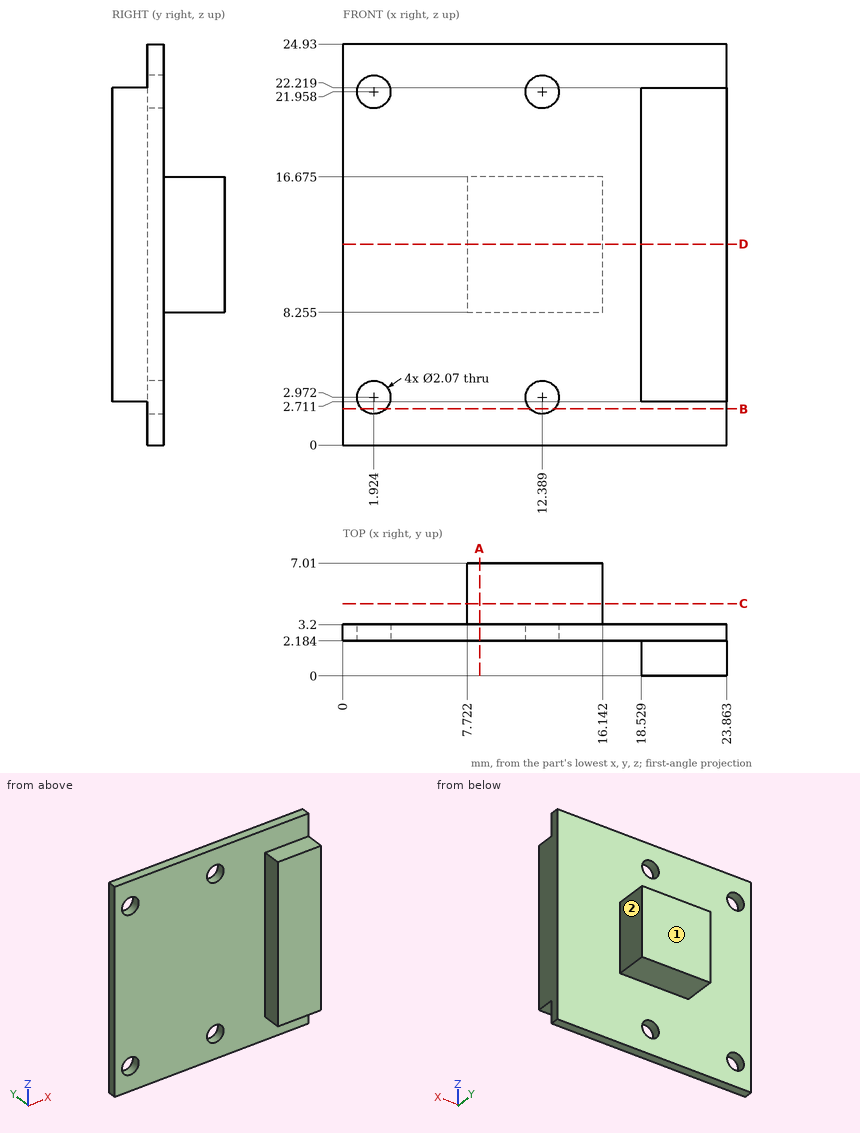
Input: dimensioned drawing with shaded views. Units: mm. Origin: part minimum x, y, z. A direction names the side the tool comes from. Coordinates: 2 decimals unless noted, no trailing zeros. Loops run counter-clockwise (first coordinate to the right, second up) from the corner with the lowest first, then second, coordinate; pieces in that order, holes last. Notation, with made-up numbers: (50.5, 33) -> (104.5, 33) arc R16 cw to (104.5, 45) -> close; hole circle Ø6 at (89.5, 6). An arc over 180 degrees is marked (long way). One line per item, written item: value. Start each with the question number.
Q1. Contact query for flat-ended pins moving along their axis: P1, Ø3, axis at x = 13, y = 5, coming from the +Z side (3 decimals); P2, Ø7, axis at x = 14, z = 8.5, coming from the -Y side; P3, Ø3, axis at y = 5, z = 10.5, coming from the -X side. Output: stop coordinate, or through.
Q2. Section query A-A, the plane x = 8.5. Return the cut outline in (y, z) (1 decimal).
Q3. Section query D-D, the plane z = 12.5. Return the cut outline in (x, y) (1 decimal).
Q4. Section query C-C, the plane y = 4.5. Return the cut outline in (x, z) (1 decimal), and give its area (3 significant figures).
Q5. Section query B-B, the plane z = 2.25. Return the cut outline in (x, y) (1 decimal).
Q6. Line query: line 1 along Z through (x, y) = (2, 3); line 2 along Y through (x, z) = (14, 1.25) (1 decimal); line 3 along X through (y, z) = (1, 4). Output: solid intervals per line, ascending.
Q7. Set-up query: the marked faces 1 and 2. Return all of +Z, -Z, +X, -X, +Y, -Y with unobstructed straight access to the full face (end or side cutting, diameter ignored); none if empty.
Results:
1. P1: z = 16.675
1. P2: y = 2.18
1. P3: x = 7.72
2. outline: (2.2, 0) -> (3.2, 0) -> (3.2, 8.3) -> (7, 8.3) -> (7, 16.7) -> (3.2, 16.7) -> (3.2, 24.9) -> (2.2, 24.9) -> close
3. outline: (0, 2.2) -> (18.5, 2.2) -> (18.5, 0) -> (23.9, 0) -> (23.9, 3.2) -> (16.1, 3.2) -> (16.1, 7) -> (7.7, 7) -> (7.7, 3.2) -> (0, 3.2) -> close
4. outline: (7.7, 8.3) -> (16.1, 8.3) -> (16.1, 16.7) -> (7.7, 16.7) -> close
4. area: 70.9 mm^2
5. outline: (0, 2.2) -> (1.2, 2.2) -> (1.2, 3.2) -> (0, 3.2) -> close; (2.7, 2.2) -> (11.6, 2.2) -> (11.6, 3.2) -> (2.7, 3.2) -> close; (13.1, 2.2) -> (23.9, 2.2) -> (23.9, 3.2) -> (13.1, 3.2) -> close
6. line 1: 0 to 1.94, 4 to 20.93, 22.99 to 24.93
6. line 2: 2.2 to 3.2
6. line 3: 18.53 to 23.86
7. face 1: +Z, -Z, +X, -X, +Y
7. face 2: +Z, -Z, +X, +Y
